Check sheet for the modelled part. Datum: model origin and axes. Units: mm. A direction names the side the tool comes from. Give positions to 0.01 mm unless a question says otherwise; leave off trailing zeros. Write each loop counter-clockwise with the first axis right and the second up, starting at its lowest first coordinate (ties: lowest second). Pieces come first, ordered by that corner, then holes. Notation, with made-up numbers: (-2.75, -39.5) -> (2.25, -39.5) arc R17 cw to (2.25, -16.5) -> close; hole circle Ø8 at (72, -16.75). An arc over 180 degrees is marked (long way). Return JSON: item names as keys, results as strings.
Autodesk Inventor part; units mm, degrees
ref_plane "YZ Plane" through (0, 0, 0) normal (1, 0, 0) x (0, 1, 0)
ref_plane "XZ Plane" through (0, 0, 0) normal (0, 1, 0) x (-1, 0, 0)
ref_plane "XY Plane" through (0, 0, 0) normal (0, 0, 1) x (1, 0, 0)
sketch "Sketch1" plane through (0, 0, 0) normal (0, 0, 1) x (1, 0, 0)
  line L0 (0.142, 0.105) -> (28.1, 0.105)
  line L1 (28.1, -1.295) -> (0.142, -1.295)
  line L2 (0.142, -1.295) -> (0.142, 0.105)
  line L3 (28.1, -1.295) -> (28.1, 0.105)
  line L4 (0.142, -1.295) -> (0.142, 0.105)
  line L5 (10.2623, 4.905) -> (13.5348, 4.905)
  line L6 (6.1805, 3.905) -> (10.2623, 3.905)
  line L7 (10.2623, 0.105) -> (6.1805, 0.105)
  line L8 (0.142, 4.905) -> (28.1, 4.905)
  line L9 (28.1, 4.905) -> (28.1, 3.905)
  line L10 (28.1, 3.905) -> (0.142, 3.905)
  line L11 (0.142, 3.905) -> (0.142, 4.905)
  line L12 (0.142, -1.295) -> (0.142, 0.105)
  line L13 (28.1, 3.905) -> (28.1, 0.105)
  line L14 (0.142, 3.905) -> (0.142, 0.105)
  line L15 (3.1, -1.295) -> (29.6, -1.295)
  line L16 (0.142, -1.295) -> (0.142, 0.105)
extrude "side" add sketch "Sketch1" along normal blind 2
sketch "Sketch2" plane through (0, 0, 0) normal (0, 0, -1) x (-1, 0, 0)
  line L0 (-26.6, -0.295) -> (-17.7228, -0.295)
  circle A0 centre (-22.1893, 1.8051) radius 1.1
  line L1 (-26.6, -0.295) -> (-17.7228, -0.295)
  line L2 (-26.6, 3.705) -> (-26.6, -0.295)
  line L3 (-17.7228, 3.705) -> (-26.6, 3.705)
  line L4 (-17.8928, -0.125) -> (-26.43, -0.125)
  line L5 (-26.43, -0.125) -> (-26.43, 3.535)
  line L6 (-26.43, 3.535) -> (-17.8928, 3.535)
  circle A1 centre (-22.1893, 1.8051) radius 1.25
  line L7 (-17.8928, 3.535) -> (-17.8928, -0.125)
  line L8 (-17.7228, -0.295) -> (-17.7228, 3.905)
  point P0 (0, 0)
  dimension "d2" = 0.17
  dimension "d4" = 0.17
  dimension "d5" = 0.17
  dimension "d6" = 2.5
  dimension "d25" = 0.17
extrude "sliding_block" add sketch "Sketch2" along normal blind 7.9 contours L4 L5 L6 L7
sketch "Sketch3" plane through (22.1893, 1.8051, 0) normal (0, 0, -1) x (-1, 0, 0)
  circle A0 centre (0, 0) radius 1.25
  point P0 (22.1893, -1.8051)
extrude "hole" cut sketch "Sketch3" against normal up to surface (2 mm away)
sketch "Sketch4" plane through (0, 0, 0) normal (0, 0, -1) x (-1, 0, 0)
  line L0 (-3.0135, 4.905) -> (-6.1805, 4.905)
  line L1 (-3.0135, 3.905) -> (-3.0135, 4.905)
  line L2 (-0.3963, 3.905) -> (-3.0135, 3.905)
  line L3 (-3.0135, 0.105) -> (-0.3963, 0.105)
  line L4 (-3.0135, -1.295) -> (-3.0135, 0.105)
  line L5 (-6.1805, -1.295) -> (-3.0135, -1.295)
  line L6 (-6.1805, 0.105) -> (-6.1805, -1.295)
  line L7 (-10.2623, 0.105) -> (-6.1805, 0.105)
  line L8 (-10.2623, -1.295) -> (-10.2623, 0.105)
  line L9 (-13.5348, -1.295) -> (-10.2623, -1.295)
  line L10 (-13.5348, 0.105) -> (-13.5348, -1.295)
  line L11 (-14, 0.105) -> (-13.5348, 0.105)
  line L12 (-14, 3.905) -> (-14, 0.105)
  line L13 (-13.5348, 3.905) -> (-14, 3.905)
  line L14 (-13.5348, 4.905) -> (-13.5348, 3.905)
  line L15 (-10.2623, 4.905) -> (-13.5348, 4.905)
  line L16 (-10.2623, 3.905) -> (-10.2623, 4.905)
  line L17 (-6.1805, 3.905) -> (-10.2623, 3.905)
  line L18 (-6.1805, 4.905) -> (-6.1805, 3.905)
  line L19 (-6.1805, -1.295) -> (-3.0135, -1.295)
  line L20 (-6.1805, 0.105) -> (-6.1805, -1.295)
  line L21 (-10.2623, 0.105) -> (-6.1805, 0.105)
  line L22 (-10.2623, -1.295) -> (-10.2623, 0.105)
  line L23 (-13.5348, -1.295) -> (-10.2623, -1.295)
  line L24 (-13.5348, 0.105) -> (-13.5348, -1.295)
  line L25 (-14, 0.105) -> (-13.5348, 0.105)
  line L26 (-14, 3.905) -> (-14, 0.105)
  line L27 (-13.5348, 3.905) -> (-14, 3.905)
  line L28 (-13.5348, 4.905) -> (-13.5348, 3.905)
  line L29 (-10.2623, 4.905) -> (-13.5348, 4.905)
  line L30 (-10.2623, 3.905) -> (-10.2623, 4.905)
  line L31 (-6.1805, 3.905) -> (-10.2623, 3.905)
  line L32 (-6.1805, 4.905) -> (-6.1805, 3.905)
  line L33 (-3.0135, 4.905) -> (-6.1805, 4.905)
  line L34 (-3.0135, 3.905) -> (-3.0135, 4.905)
  line L35 (-0.3963, 3.905) -> (-3.0135, 3.905)
  line L36 (-0.3963, 0.105) -> (-0.3963, 3.905)
  line L37 (-3.0135, 0.105) -> (-0.3963, 0.105)
  line L38 (-3.0135, -1.295) -> (-3.0135, 0.105)
  line L39 (-0.3963, 0.105) -> (-0.142, 0.105)
  line L40 (-0.142, 4.905) -> (-0.142, -1.295)
  line L41 (-0.3963, 3.905) -> (-0.142, 3.905)
  line L42 (-0.142, 3.905) -> (-0.142, 0.105)
extrude "alignment_cut" cut sketch "Sketch4" against normal blind 0.5
sketch "Sketch5" plane through (0, 0, 2) normal (0, 0, 1) x (1, 0, 0)
  line L0 (22.1893, 4.1145) -> (24.1893, 2.9598)
  line L1 (24.1893, 2.9598) -> (24.1893, 0.6504)
  line L2 (24.1893, 0.6504) -> (22.1893, -0.5043)
  line L3 (22.1893, -0.5043) -> (20.1893, 0.6504)
  line L4 (20.1893, 0.6504) -> (20.1893, 2.9598)
  line L5 (20.1893, 2.9598) -> (22.1893, 4.1145)
  circle A0 centre (22.1893, 1.8051) radius 1.25
  point P0 (0, 0)
  dimension "d19" = 4
sketch "Sketch6" plane through (0, 0, 0) normal (0, 0, -1) x (-1, 0, 0)
  line L0 (-0.142, -1.295) -> (-28.1, -1.295)
  line L1 (-0.142, -1.295) -> (-28.1, -1.295)
  line L2 (-28.1, 4.905) -> (-0.142, 4.905)
  line L3 (-28.1, 4.905) -> (-13.5348, 4.905)
  line L4 (-3.0135, 3.905) -> (-3.0135, 4.905)
  line L5 (-0.142, 4.905) -> (-3.0135, 4.905)
  line L6 (-0.142, 3.905) -> (-3.0135, 3.905)
  line L7 (-0.142, -1.295) -> (-3.0135, -1.295)
  line L8 (-13.5348, -1.295) -> (-13.5348, 0.105)
  line L9 (-13.5348, 0.105) -> (-14, 0.105)
  line L10 (-14, 0.105) -> (-14, 3.905)
  line L11 (-14, 3.905) -> (-13.5348, 3.905)
  line L12 (-13.5348, 3.905) -> (-13.5348, 4.905)
  line L13 (-13.5348, -1.295) -> (-28.1, -1.295)
  line L14 (-10.2623, 0.105) -> (-10.2623, -1.295)
  line L15 (-6.1805, -1.295) -> (-10.2623, -1.295)
  line L16 (-6.1805, -1.295) -> (-6.1805, 0.105)
  line L17 (-6.1805, 0.105) -> (-10.2623, 0.105)
  line L18 (-3.0135, 0.105) -> (-3.0135, -1.295)
  line L19 (-0.142, 4.905) -> (-0.142, 3.905)
  line L20 (-3.0135, 4.905) -> (-3.0135, 3.905)
  line L21 (-10.2623, 4.905) -> (-10.2623, 3.905)
  line L22 (-10.2623, 3.905) -> (-6.1805, 3.905)
  line L23 (-6.1805, 3.905) -> (-6.1805, 4.905)
  line L24 (-3.0135, 4.905) -> (-0.142, 4.905)
  line L25 (-10.2623, 4.905) -> (-6.1805, 4.905)
  line L26 (-28.1, -1.295) -> (-28.1, 4.905)
  line L27 (-26.43, 3.535) -> (-17.8928, 3.535)
  line L28 (-17.8928, 3.535) -> (-17.8928, -0.125)
  line L29 (-17.8928, -0.125) -> (-26.43, -0.125)
  line L30 (-26.43, -0.125) -> (-26.43, 3.535)
  line L31 (-0.142, 3.905) -> (-0.142, 4.905)
  line L32 (-0.142, 0.105) -> (-0.142, -1.295)
  line L33 (-0.142, 0.105) -> (-3.0135, 0.105)
  line L34 (-3.0135, 3.905) -> (-0.142, 3.905)
  point P0 (-0.1, 0.105)
  point P1 (-0.1, 3.905)
extrude "probe_slot" add sketch "Sketch6" along normal blind 0.3 contours L0 L18 L33 L32 | L2 L19 L6 L4
extrude "nut_slot" cut sketch "Sketch5" against normal blind 1.5 contours L0 L1 L2 L3 L4 L5 | A0
fillet "Fillet3" radius 2.3 1 edges at (0.142, 1.805, 2)
equation "\"d4\" = d2"
equation "\"d5\" = d2"
equation "\"d25\" = d2"
properties part number "stereotax_side"
(1) Cross-section at C-C on x = 25.75. Enter the section's corners in (y, z) (3 decimals), then the cut area to 3 significant figures.
Reply:
{"outline": "(-1.295, 0) -> (-0.125, 0) -> (-0.125, -7.9) -> (3.535, -7.9) -> (3.535, 0) -> (4.905, 0) -> (4.905, 2) -> (-1.295, 2) -> close", "area": "41.3 mm^2"}
(2) Cross-section at B-B on x = 21.75. Enter the section's corners in (y, z) (3 decimals), then the cut area to 3 significant figures.
Reply:
{"outline": "(-1.295, 0) -> (-0.125, 0) -> (-0.125, -7.9) -> (0.635, -7.9) -> (0.635, 0.5) -> (-0.251, 0.5) -> (-0.251, 2) -> (-1.295, 2) -> close; (2.975, -7.9) -> (3.535, -7.9) -> (3.535, 0) -> (4.905, 0) -> (4.905, 2) -> (3.861, 2) -> (3.861, 0.5) -> (2.975, 0.5) -> close", "area": "15.5 mm^2"}
(3) Release check for a two-part mould opening along X. For faces 1 (the flat face through (21, 1, -7.9)), 2 (the flat face through (7, 2, 0.5)), 3 (the flat face through (26.43, 2, -4)) record: pulls with the +X half, pulls with the -X half, needs draft (parallel to the pull), parting line crosses it, or undercut.
Reply:
{"face 1": "needs draft", "face 2": "undercut", "face 3": "pulls with the +X half"}
(4) Cross-section at D-D on z = 1.25. Enter the section's corners in (x, y) (1 decimal).
Reply:
{"outline": "(0.7, -1.3) -> (28.1, -1.3) -> (28.1, 4.9) -> (0.7, 4.9) -> close; hole (20.2, 0.7) -> (22.2, -0.5) -> (24.2, 0.7) -> (24.2, 3) -> (22.2, 4.1) -> (20.2, 3) -> close"}
(5) Depth check by flat-ended pin: pin 1 Ø1 at (x, z) = (19, -5) entering from -Y (3 decimals); pin 2 Ø1.1 at (y, z) = (2.5, -4.5) entering from -X; pin 3 Ø1.2 at (y, z) = (2, 1.5) entering from -X. Enter the tip coordinate at first touch or a pass-through.
Reply:
{"pin 1": "y = -0.125", "pin 2": "x = 17.89", "pin 3": "x = 0.48"}
(6) Cross-section at A-A on y = 2.25. Enter the section's corners in (x, z), then the cut area to 3 significant figures.
Reply:
{"outline": "(0.29, 0.5) -> (14, 0.5) -> (14, 0) -> (17.89, 0) -> (17.89, -7.9) -> (21.02, -7.9) -> (21.02, 0.5) -> (20.19, 0.5) -> (20.19, 2) -> (2.44, 2) arc R2.3 ccw to start; (23.36, -7.9) -> (26.43, -7.9) -> (26.43, 0) -> (28.1, 0) -> (28.1, 2) -> (24.19, 2) -> (24.19, 0.5) -> (23.36, 0.5) -> close", "area": "89.7 mm^2"}
(7) Thickness scan on L1, parallel to Y at x = 22.25, z = 0.25 (3 decimals); L2, parallel to X at y = 1.75, z = -2.5; L3, parallel to Z at x = 17.5, y = 4.5. Record the ranges inside material, lowest first.
Reply:
{"L1": "-1.295 to 0.557, 3.054 to 4.905", "L2": "17.89 to 20.94, 23.44 to 26.43", "L3": "0 to 2"}
(8) Set-up check for faces 4 (the flat face through (1.6, 4.4, -0.3)), 5 (the flat face through (8.2, 4.4, 0)), 6 (the flat face through (8, -1, 0)), 7 (the flat face through (23.2, 0.08, 1.26)): record each of +Z, -Z, +X, -X, +Y, -Y from which the full face is reachable in a straight line by a thin tool's end or side.
Reply:
{"face 4": "-Z, +X, -X, +Y, -Y", "face 5": "-Z, +X, +Y, -Y", "face 6": "-Z, +Y, -Y", "face 7": "+Z"}
